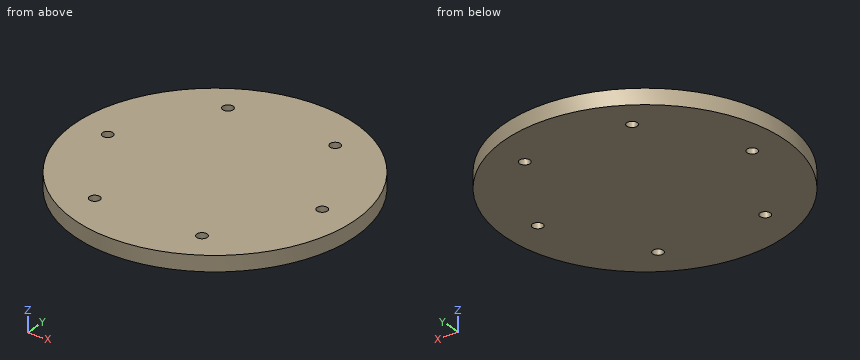
```python
from build123d import *

# Parameters (mm, degrees)
F0_R            = 46.355
F1_DEPTH        = 5.08
F4_D            = 3.4544
F4_COPIES_COUNT = 6


# Not quite as in the source:
# - a pattern or mirror of a feature is missing from the dataset's text; its kind, count and spacing are read off the source's solid


with BuildPart() as f1:
    # F0 (on Top) → F1 (new body)
    with BuildSketch(Plane.XY):
        Circle(F0_R)
    extrude(amount=F1_DEPTH)

    # F4 (through all)
    with Locations(Plane(origin=(0, 0, 0), x_dir=(1, 0, 0), z_dir=(0, 0, -1))):
        with Locations((35.56, 0)):
            f4 = Hole(F4_D / 2)

    # F4_copies: F4 ×6 about axis
    f4_copies_axis = Axis((0, 0, 0), (0, 0, 1))
    for i in range(1, F4_COPIES_COUNT):
        add(f4.rotate(f4_copies_axis, i * 360 / F4_COPIES_COUNT), mode=Mode.SUBTRACT)


solid = f1.part
```
Check sheet for the modelled part. Datum: model origin and axes. Units: mm. Round coordinates to 2 decimals unless told otherwise and drop trailing zeros. Order: outer loops, then holes, each group sorted by start corner. A loop starts at its lowest first (then second) coordinate and runs counter-clockwise, first axis right, second up. Notation, with made-up numbers: (48.5, -19) - (100.5, -19) arc R18 ccw to (100.5, -3) - close; hole circle Ø7 at (21, -31). An arc over 180 degrees is marked (long way). Answer as CSV lines item,"result". Start each with the question number.
1) Section check B-B (x = 35.56). Record the cut outline in (y, z), then the cut area to 3 significant figures.
2) Depth check by flat-ended pin: pin 1 (1.5 mm diameter, centred on x = 16.5, z = 2.5, fed in from -Y); pin 2 (3 mm diameter, centred on x = -17.78, y = 30.8, fed in from +Z); pin 3 (3 mm diameter, centred on x = 15, z = 2.5, fed in from -Y); pin 4 (2 mm diameter, centred on x = 3.5, z = 3, fed in from +Y). Enter the tip coordinate at first touch or a pass-through.
3) Section check A-A (y = 0). Record the cut outline in (x, z) (3 decimals).
4) Section check D-D (x = -10.5). Record the cut outline in (y, z).
5) Scan lines: probe 1 along Y at (x, z) = (17.78, 3.9); probe 2 along Y at (x, z) = (35.56, 3.75); probe 3 along Y at (x, z) = (0, 0.6) (3 decimals). Record each from-to range of solid material in increasing order.
6) Section check C-C (z = 4.1). Record the cut outline in (x, y) (3 decimals).
Determined:
1,outline,"(-29.74, 0) - (-1.73, 0) - (-1.73, 5.08) - (-29.74, 5.08) - close; (1.73, 0) - (29.74, 0) - (29.74, 5.08) - (1.73, 5.08) - close"
1,area,"285 mm^2"
2,pin 1,"y = -43.6"
2,pin 2,"through"
2,pin 3,"y = -44.35"
2,pin 4,"y = 46.29"
3,outline,"(-46.355, 0) - (-37.287, 0) - (-37.287, 5.08) - (-46.355, 5.08) - close; (-33.833, 0) - (33.833, 0) - (33.833, 5.08) - (-33.833, 5.08) - close; (37.287, 0) - (46.355, 0) - (46.355, 5.08) - (37.287, 5.08) - close"
4,outline,"(-45.15, 0) - (45.15, 0) - (45.15, 5.08) - (-45.15, 5.08) - close"
5,probe 1,"-42.81 to -32.52, -29.07 to 29.07, 32.52 to 42.81"
5,probe 2,"-29.74 to -1.73, 1.73 to 29.74"
5,probe 3,"-46.355 to 46.355"
6,outline,"circle Ø92.71 at (0, 0); hole circle Ø3.454 at (-35.56, 0); hole circle Ø3.454 at (-17.78, -30.796); hole circle Ø3.454 at (-17.78, 30.796); hole circle Ø3.454 at (17.78, -30.796); hole circle Ø3.454 at (17.78, 30.796); hole circle Ø3.454 at (35.56, 0)"
